```python
from build123d import *

# Parameters (mm, degrees)
SKETCH1_W           = 101.6
SKETCH1_H           = 139.7
BOSS_EXTRUDE1_DEPTH = 19.05


with BuildPart() as part:
    # Sketch1 → Boss-Extrude1 (new body)
    with BuildSketch(Plane(origin=(0, 0, 0), x_dir=(1, 0, 0), z_dir=(0, 1, 0))):
        Rectangle(SKETCH1_W, SKETCH1_H)
    extrude(amount=BOSS_EXTRUDE1_DEPTH)

    # Sketch2 → 3/4 (0.75) Diameter Hole1 (revolve, cut)
    with BuildSketch(Plane(origin=(-25.4, 19.05, -50.8), x_dir=(0, 0, 1), z_dir=(1, 0, 0))):
        Polygon((0, 0), (0, 24.773197396), (9.525, 19.05), (9.525, 0), align=None)
    f_3_4_0_75_diameter_hole1 = revolve(axis=Axis((-25.4, 25.4, -50.8), (0, -1, 0)), mode=Mode.SUBTRACT)

    # Mirror1: 3/4 (0.75) Diameter Hole1 across plane
    add(f_3_4_0_75_diameter_hole1.mirror(Plane.XY), mode=Mode.SUBTRACT)

    # Mirror4: 3/4 (0.75) Diameter Hole1 across plane
    add(f_3_4_0_75_diameter_hole1.mirror(Plane(origin=(0, 0, 0), x_dir=(0, 0, 1), z_dir=(1, 0, 0))), mode=Mode.SUBTRACT)

    # Mirror4 copy 1 sketch → Mirror4 copy 1 (revolve, cut)
    with BuildSketch(Plane(origin=(25.4, 19.05, 50.8), x_dir=(0, 0, -1), z_dir=(-1, 0, 0))):
        Polygon((0, 0), (0, 24.773197396), (9.525, 19.05), (9.525, 0), align=None)
    revolve(axis=Axis((25.4, 25.4, 50.8), (0, -1, 0)), mode=Mode.SUBTRACT)

    # Sketch4 → 1/4 (0.25) Diameter Hole1 (revolve, cut)
    with BuildSketch(Plane(origin=(25.4, 9.525, -69.85), x_dir=(0, 1, 0), z_dir=(1, 0, 0))):
        Polygon((0, 0), (0, 20.957732465), (3.175, 19.05), (3.175, 0), align=None)
    f_1_4_0_25_diameter_hole1 = revolve(axis=Axis((25.4, 9.525, -76.2), (0, 0, 1)), mode=Mode.SUBTRACT)

    # Mirror5: 1/4 (0.25) Diameter Hole1 across plane
    add(f_1_4_0_25_diameter_hole1.mirror(Plane.XY), mode=Mode.SUBTRACT)

    # Mirror10: 1/4 (0.25) Diameter Hole1 across plane
    add(f_1_4_0_25_diameter_hole1.mirror(Plane(origin=(0, 0, 0), x_dir=(0, 0, 1), z_dir=(1, 0, 0))), mode=Mode.SUBTRACT)

    # Mirror10 copy 1 sketch → Mirror10 copy 1 (revolve, cut)
    with BuildSketch(Plane(origin=(-25.4, 9.525, 69.85), x_dir=(0, 1, 0), z_dir=(-1, 0, 0))):
        Polygon((0, 0), (0, 20.957732465), (3.175, 19.05), (3.175, 0), align=None)
    revolve(axis=Axis((-25.4, 9.525, 76.2), (0, 0, -1)), mode=Mode.SUBTRACT)


solid = part.part
```
Model file for the job. Use its own axes, mm. A direction names the side the tool comes from. Give positions to 0.01 mm unless a question says otherwise; leave off trailing zeros. Write each loop counter-clockwise with the first axis right and the second up, starting at its lowest first coordinate (ties: lowest second). Pieces come first, ordered by that corner, then holes. Notation, with made-up numbers: (34, 18) -> (93, 18) arc R10 ccw to (93, 37) -> close; hole circle Ø10 at (16.5, -5). An arc over 180 degrees is marked (long way). Use CSV: the item, a comma, the result in double quotes. Start each with the question number.
1) Two-plate mould, pull along Z, no slides. Class faces 1 (the flat face through (50.8, 9, 1)), 2 (the cylindrical face through (-21.75, 9.66, 42)), 3 (the flat face through (-1, 9, 69.85)), 4 (the flat face through (-1, 9, -69.85)): released by +Z, released by -Z, zero draft, split by the parting line, or undercut.
2) Cut at B-B on z = 51. List the corners of the cut face in (x, y), plus the area to 3 significant figures.
3) Cut at D-D on y = 8. List the corners of the cut face in (x, z) (3 decimals), plus the area to 3 significant figures.
4) Tool access for faces 5 (the flat face through (-50.8, 9, 1)), 6 (the cylindrical face through (22.72, 11.23, 64.89)), 7 (the cylindrical face through (-22.72, 11.23, -64.89)): list every direction of +Z, -Z, +X, -X, +Y, -Y with a clear straight run to the whole face (end or side of a thin tool).
5) Pin check, flat tips, straight feed: P1, Ø5.5, axis at x = 25.4, y = 9.525, coming from the +Z side; P2, Ø15, axis at x = -25.4, z = -50.8, coming from the -Y side (3 decimals); P3, Ø5, axis at x = 25.4, y = 9.525, coming from the -Z side; P4, Ø4, axis at x = -25.4, y = 9.525, coming from the -Z side. Stop position of each tip, or through.
6) Cut at A-A on y = 14.5. List the corners of the cut face in (x, z) (3 decimals).
7) Cut at C-C on x = 25.4. List the corners of the cut face in (y, z) (3 decimals), plus the area to 3 significant figures.
8) Drill centre lines: L1, parallel to X at y = 6.25, z = 50.8 (3 decimals); L2, parallel to Z at x = -17, y = 10; L3, parallel to Y at x = 25.4, z = -66.25. Where is each one in solid material? Low to high.
Final values:
1,face 1,"zero draft"
1,face 2,"undercut"
1,face 3,"released by +Z"
1,face 4,"released by -Z"
2,outline,"(-50.8, 0) -> (-34.92, 0) -> (-34.92, 19.05) -> (-50.8, 19.05) -> close; (-15.88, 0) -> (15.88, 0) -> (15.88, 19.05) -> (-15.88, 19.05) -> close; (34.92, 0) -> (50.8, 0) -> (50.8, 19.05) -> (34.92, 19.05) -> close"
2,area,"1,210 mm2"
3,outline,"(-50.8, -69.85) -> (-28.185, -69.85) -> (-28.185, -59.909) arc R9.525 cw (long way) to (-22.615, -59.909) -> (-22.615, -69.85) -> (22.615, -69.85) -> (22.615, -59.909) arc R9.525 cw (long way) to (28.185, -59.909) -> (28.185, -69.85) -> (50.8, -69.85) -> (50.8, 69.85) -> (28.185, 69.85) -> (28.185, 59.909) arc R9.525 cw (long way) to (22.615, 59.909) -> (22.615, 69.85) -> (-22.615, 69.85) -> (-22.615, 59.909) arc R9.525 cw (long way) to (-28.185, 59.909) -> (-28.185, 69.85) -> (-50.8, 69.85) -> close"
3,area,"12,800 mm2"
4,face 5,"+Z, -Z, -X, +Y, -Y"
4,face 6,"+Z"
4,face 7,"-Z"
5,P1,"stops at z = 41.68"
5,P2,"passes through"
5,P3,"stops at z = -41.61"
5,P4,"stops at z = -41.49"
6,outline,"(-50.8, -69.85) -> (50.8, -69.85) -> (50.8, 69.85) -> (-50.8, 69.85) -> close; hole circle Ø19.05 at (-25.4, -50.8); hole circle Ø19.05 at (-25.4, 50.8); hole circle Ø19.05 at (25.4, -50.8); hole circle Ø19.05 at (25.4, 50.8)"
7,outline,"(0, -69.85) -> (6.35, -69.85) -> (6.35, -60.325) -> (0, -60.325) -> close; (0, -41.275) -> (19.05, -41.275) -> (19.05, 41.275) -> (0, 41.275) -> close; (0, 60.325) -> (6.35, 60.325) -> (6.35, 69.85) -> (0, 69.85) -> close; (12.7, -69.85) -> (19.05, -69.85) -> (19.05, -60.325) -> (12.7, -60.325) -> close; (12.7, 60.325) -> (19.05, 60.325) -> (19.05, 69.85) -> (12.7, 69.85) -> close"
7,area,"1,810 mm2"
8,L1,"x = -50.8 to -34.925, -15.875 to 15.875, 34.925 to 50.8"
8,L2,"z = -69.85 to -55.29, -46.31 to 46.31, 55.29 to 69.85"
8,L3,"y = 0 to 6.35, 12.7 to 19.05"
